Autodesk Inventor part; units mm, degrees
ref_plane "YZ Plane" through (0, 0, 0) normal (1, 0, 0) x (0, 1, 0)
ref_plane "XZ Plane" through (0, 0, 0) normal (0, 1, 0) x (-1, 0, 0)
ref_plane "XY Plane" through (0, 0, 0) normal (0, 0, 1) x (1, 0, 0)
sketch "スケッチ1" plane through (0, 0, 0) normal (0, 0, 1) x (1, 0, 0)
  circle A0 centre (0, 0) radius 3
  dimension "d0" = 6
extrude "押し出し1" add sketch "スケッチ1" along normal blind 35
sketch "スケッチ2" plane through (0, 0, 35) normal (0, 0, 1) x (1, 0, 0)
  circle A0 centre (0, 0) radius 1.4
  dimension "d3" = 2.8
extrude "押し出し2" cut sketch "スケッチ2" against normal blind 6
sketch "スケッチ3" plane through (0, 0, 0) normal (0, 0, -1) x (-1, 0, 0)
  circle A0 centre (0, 0) radius 1.4
  circle A1 centre (0, 0) radius 1.4
extrude "押し出し3" cut sketch "スケッチ3" against normal blind 6
properties part number "34mm" material "アルミニウム 6061"
Check sheet for the modelled part. Datum: model origin and axes. Units: mm. Coordinates: 2 decimals unless noted, no trailing zeros. Write each loop counter-clockwise with the first axis right and the second up, starting at its lowest first coordinate (ties: lowest second). Pieces come first, ordered by that corner, then holes.
Item 1: Mould release check, pull along Y, two halves, no side actions. Record for faces 1 (the face through (0, 0, 29)), 2 (the face through (-3, 0, 17)), 3 (the face through (-1.4, 0.06, 32.04)): released by +Y, released by -Y, zero draft, split by the parting line, or undercut.
Numbers:
face 1: undercut
face 2: split by the parting line
face 3: undercut
Item 2: Cross-section at A-A on x = 0. Record the boundary of the cut face in (y, z).
Numbers:
outline: (-3, 0) - (-1.4, 0) - (-1.4, 6) - (1.4, 6) - (1.4, 0) - (3, 0) - (3, 35) - (1.4, 35) - (1.4, 29) - (-1.4, 29) - (-1.4, 35) - (-3, 35) - close
Item 3: Depth check by flat-ended pin: pin 1 Ø2.5 at (x, y) = (0, 0) entering from +Z; pin 2 Ø1.7 at (x, y) = (0, 0) entering from -Z; pin 3 Ø2 at (x, z) = (2.5, 25) entering from +Y. Enter the tip coordinate at first touch or a pass-through.
Numbers:
pin 1: stops at z = 29
pin 2: stops at z = 6
pin 3: stops at y = 2.6
Item 4: Cross-section at C-C on z = 30.5. Record the boundary of the cut face in (x, y), then the cut area to 3 significant figures.
Numbers:
outline: circle Ø6 at (0, 0); hole circle Ø2.8 at (0, 0)
area: 22.1 mm2
Item 5: Scan lines: probe 1 along Y at (x, z) = (0, 33.5); probe 2 along Z at (x, y) = (-0.3, -0.85); probe 3 along X at (y, z) = (0.25, 22). Record each from-to range of solid material in increasing order.
Numbers:
probe 1: y = -3 to -1.4, 1.4 to 3
probe 2: z = 6 to 29
probe 3: x = -2.99 to 2.99
Item 6: Cross-section at D-D on z = 13. Record the boundary of the cut face in (x, y).
Numbers:
outline: circle Ø6 at (0, 0)
